Input: part model. Units: mm. Frame: model coordinates. Round coordinates to 2 decimals unless told otherwise and drop trailing zeros. Loops run counter-clockwise (first coordinate to the right, second up) from the corner with the lowest first, then second, coordinate; pieces in that order, holes last. Notation, with made-up numbers: (18, 49) -> (69, 49) arc R24 ccw to (69, 76) -> close; hole circle Ø8 at (40, 17). An arc over 180 degrees is marked (long way). Answer as a JSON object with one key per item and string values. Group by question number.
Item 1: Section query C-C on x = 96.5. Return loops of the section in (y, z) (3 decimals).
Item 2: Section query B-B on y = 31. Return loops of the section in (x, z) (3 decimals).
Item 3: Section query A-A on y = 21. Return loops of the section in (x, z) (3 decimals), and give its area (3 significant figures).
Item 4: Section query D-D on z = 2.05. Return loops of the section in (x, y) (1 decimal).
Item 5: Material intervals for line 1 (X direction, y = 16.5, z = 0.55); line 2 (Y direction, x = 99.5, z = 1.05); line 3 (Y direction, x = 96, z = 1.75), sorted ascending. Write a range as [from, to].
Item 6: Pin query (flat end, axial travel): pin 1 (1.6 mm diameter, centred on x = 11.5, z = 2, fed in from -Y); pin 2 (1 mm diameter, centred on y = 28, z = 1, fed in from +X). Return the tip coordinate at first contact, or that it passes through.
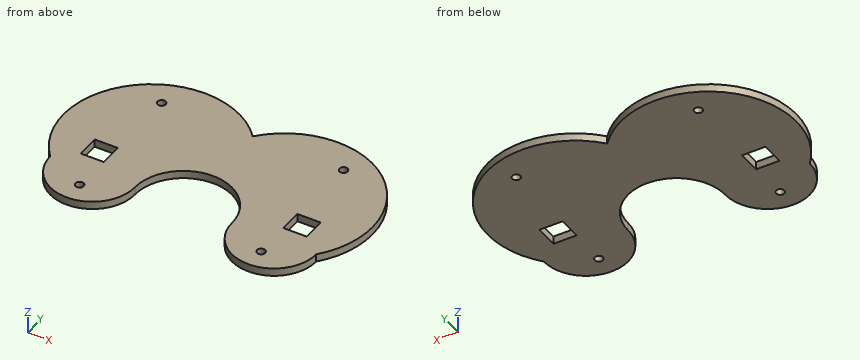
from build123d import *

# Parameters (mm, degrees)
BOSS_EXTRUDE1_DEPTH = 3.175
SKETCH2_R           = 1.6637
CUT_EXTRUDE1_DEPTH  = 3.175
SKETCH3_W           = 9.398
SKETCH3_H           = 9.398
CUT_EXTRUDE2_DEPTH  = 3.175


with BuildPart() as part:
    # Sketch1 → Boss-Extrude1 (new body)
    with BuildSketch(Plane.XY):
        with BuildLine():
            ThreePointArc((34.288648696, 17.145), (17.143648696, 0), (-0.001351304, 17.145))
            ThreePointArc((-0.001351304, 17.145), (3.871238611, 67.363724589), (54.080955836, 63.376050056))
            ThreePointArc((54.080955836, 63.376050056), (104.238720612, 67.087510011), (107.950180567, 16.929745235))
            ThreePointArc((107.950180567, 16.929745235), (90.72699247, -0.107108433), (73.66126725, 17.087472513))
            ThreePointArc((73.66126725, 17.087472513), (54.003763774, 36.831330291), (34.288648696, 17.145))
        make_face()
    extrude(amount=BOSS_EXTRUDE1_DEPTH)

    # Sketch2 → Cut-Extrude1 (cut)
    with BuildSketch(Plane.XY.offset(3.175)):
        with Locations((17.143648696, 8.5725)):
            Circle(SKETCH2_R)
        with Locations((90.766339889, 8.438225181)):
            Circle(SKETCH2_R)
        with Locations((17.143648696, 63.376050056)):
            Circle(SKETCH2_R)
        with Locations((91.017638263, 63.161224448)):
            Circle(SKETCH2_R)
    extrude(amount=-CUT_EXTRUDE1_DEPTH, mode=Mode.SUBTRACT)

    # Sketch3 → Cut-Extrude2 (cut)
    with BuildSketch(Plane.XY.offset(3.175)):
        with Locations((12.850394595, 28.73375)):
            Rectangle(SKETCH3_W, SKETCH3_H)
        with Locations((95.120347818, 28.620185079)):
            Rectangle(SKETCH3_W, SKETCH3_H)
    extrude(amount=-CUT_EXTRUDE2_DEPTH, mode=Mode.SUBTRACT)


solid = part.part
Solved:
{
 "1": {"outline": "(0.866, 0) -> (23.921, 0) -> (23.921, 3.175) -> (0.866, 3.175) -> close; (33.319, 0) -> (72.169, 0) -> (72.169, 3.175) -> (33.319, 3.175) -> close"},
 "2": {"outline": "(-7.345, 0) -> (8.151, 0) -> (8.151, 3.175) -> (-7.345, 3.175) -> close; (17.549, 0) -> (39.99, 0) -> (39.99, 3.175) -> (17.549, 3.175) -> close; (67.96, 0) -> (90.421, 0) -> (90.421, 3.175) -> (67.96, 3.175) -> close; (99.819, 0) -> (115.381, 0) -> (115.381, 3.175) -> (99.819, 3.175) -> close"},
 "3": {"outline": "(-2.883, 0) -> (34.67, 0) -> (34.67, 3.175) -> (-2.883, 3.175) -> close; (73.28, 0) -> (110.981, 0) -> (110.981, 3.175) -> (73.28, 3.175) -> close", "area": "239 mm²"},
 "4": {"outline": "(0, 17.1) arc R17.1 ccw to (34.3, 17.1) arc R19.7 cw to (73.7, 17.1) arc R17.1 ccw to (108, 16.9) arc R35.6 ccw to (54.1, 63.4) arc R35.6 ccw to start; hole (8.2, 24) -> (17.5, 24) -> (17.5, 33.4) -> (8.2, 33.4) -> close; hole circle Ø3.3 at (17.1, 8.6); hole circle Ø3.3 at (17.1, 63.4); hole circle Ø3.3 at (90.8, 8.4); hole circle Ø3.3 at (91, 63.2); hole (90.4, 23.9) -> (99.8, 23.9) -> (99.8, 33.3) -> (90.4, 33.3) -> close"},
 "5": {"line 1": "[0.01, 34.28], [73.67, 107.94]", "line 2": "[2.26, 23.92], [33.32, 70.54]", "line 3": "[0.7, 23.92], [33.32, 72.41]"},
 "6": {"pin 1": "y = 0.7", "pin 2": "x = 114.62"}
}
